from build123d import *

# Parameters (mm, degrees)
F1_DEPTH = 76.2
F3_DEPTH = 27.94
F4_R     = 10.16
F5_DEPTH = 76.201
F6_W     = 5.08
F6_H     = 76.2
F7_DEPTH = 10.16
F8_R     = 14.139528
F9_DEPTH = 25.4


with BuildPart() as f1:
    # F0 (on Right) → F1 (new body)
    with BuildSketch(Plane.YZ):
        Polygon((-76.2, 35.56), (-76.2, 0), (35.56, 0), (71.12, 35.56), (71.12, 71.12), (35.56, 71.12), (0, 35.56), align=None)
    extrude(amount=F1_DEPTH)

    # F2 (on face) → F3 (cut)
    with BuildSketch(Plane.XY.offset(71.12)):
        with BuildLine():
            Line((60.96, 60.96), (15.24, 60.96))
            ThreePointArc((15.24, 60.96), (7.62, 53.34), (15.24, 45.72))
            Line((15.24, 45.72), (60.96, 45.72))
            ThreePointArc((60.96, 45.72), (68.58, 53.34), (60.96, 60.96))
        make_face()
    extrude(amount=-F3_DEPTH, mode=Mode.SUBTRACT)

    # F4 (on face) → F5 (cut, through all)
    with BuildSketch(Plane.YZ.offset(76.2)):
        with Locations((17.78, 20.32)):
            Circle(F4_R)
    extrude(amount=-F5_DEPTH, mode=Mode.SUBTRACT)

    # F6 (on face) → F7 (cut)
    with BuildSketch(Plane.XY.offset(35.56)):
        with Locations((36.052045, -38.1)):
            Rectangle(F6_W, F6_H)
    extrude(amount=-F7_DEPTH, mode=Mode.SUBTRACT)

    # F8 (on face) → F9 (cut)
    with BuildSketch(Plane.XY.offset(35.56)):
        with Locations((36.461484, -37.369102)):
            Circle(F8_R)
    extrude(amount=-F9_DEPTH, mode=Mode.SUBTRACT)


solid = f1.part
The listing builds one solid part. Answer for the finished solid, in the listing's coordinates (mm). A direction names the side the tool comes from. Coordinates: 2 decimals unless noted, no trailing zeros. Order: outer loops, then holes, each group sorted by start corner. A loop starts at its lowest first (then second) coordinate and runs counter-clockwise, first axis right, second up. Notation, with made-up numbers: (20, 18) -> (26, 18) arc R30 ccw to (26, 57) -> close; hole circle Ø2 at (17.5, 35.25). An arc over 180 degrees is marked (long way). Answer in a Markdown table with one row per item. Add a question column.
Item 1: Find section C-C (z = 20.32). Write down the section's boundary in (x, y).
Item 2: Each of these flat-tipped pins is pushed along its axis until it touches: P1, Ø5.5, axis at x = 35.5, y = -17.5, coming from the +Z side; P2, Ø2.5, axis at x = 36, y = -60.5, coming from the +Z side; P3, Ø2, axis at x = 13.5, z = 23.5, coming from the +Y side. Where does it stop, or does it pass through?
Item 3: Find section D-D (x = 20). Write down the section's boundary in (y, z), then the cut area to 3 significant figures.
Item 4: Which of the six approach directions +Z, -Z, +X, -X, +Y, -Y give full straight-line access (tool end or side, diameter ignored) to faces 5 (the face through (37.57, 53.09, 17.53)), 6 (the face through (38, -21, 0)), 7 (the face through (33.512, -64, 31)), 8 (the face through (36, -37, 10.16)), 9 (the face through (17, -38, 35.56))?
Item 5: Find section B-B (z = 49). Write down the section's boundary in (x, y), then the cut area to 3 significant figures.
Item 6: Find the intervals of material crossed by L1, parallel to Y at x = 36.5, z = 25; L2, parallel to Y at x = 39.5, z = 22.5; L3, parallel to X at y = -9, z = 27, in increasing order. Write a range as from..to.
Item 7: Find section A-A (y = 17.78). Write down the section's boundary in (x, z).
Item 8: Determine the mould class of faces 1 (the face through (33.512, -12, 31)), 2 (the face through (38, -76.2, 18)), 3 (the face through (76.2, -4, 28)), 4 (the face through (0, -4, 28)) for opening direction X: +X half, -X half, draft (parallel to the pull), parting line (faces both ways), or undercut.
Result set:
| question | item | result |
|---|---|---|
| 1 | outline | (0, -76.2) -> (76.2, -76.2) -> (76.2, 7.62) -> (0, 7.62) -> close; (0, 27.94) -> (76.2, 27.94) -> (76.2, 55.88) -> (0, 55.88) -> close; hole circle Ø28.28 at (36.46, -37.37) |
| 2 | P1 | stops at z = 35.56 |
| 2 | P2 | stops at z = 25.4 |
| 2 | P3 | stops at y = 60.06 |
| 3 | outline | (-76.2, 0) -> (35.56, 0) -> (71.12, 35.56) -> (71.12, 71.12) -> (60.96, 71.12) -> (60.96, 43.18) -> (45.72, 43.18) -> (45.72, 71.12) -> (35.56, 71.12) -> (0, 35.56) -> (-76.2, 35.56) -> close; hole circle Ø20.32 at (17.78, 20.32) |
| 3 | area | 5,750 mm² |
| 4 | face 5 | -Z, +X, -X, +Y |
| 4 | face 6 | -Z, +X, -X, +Y, -Y |
| 4 | face 7 | +Z, -Y |
| 4 | face 8 | +Z |
| 4 | face 9 | +Z, +X, -X, -Y |
| 5 | outline | (0, 13.44) -> (76.2, 13.44) -> (76.2, 71.12) -> (0, 71.12) -> close; hole (15.24, 45.72) -> (60.96, 45.72) arc R7.62 ccw to (60.96, 60.96) -> (15.24, 60.96) arc R7.62 ccw to start |
| 5 | area | 3,520 mm² |
| 6 | L1 | y = -76.2..-51.51, -23.23..8.76, 26.8..60.56 |
| 6 | L2 | y = -76.2..-51.18, -23.56..7.86, 27.7..58.06 |
| 6 | L3 | x = 0..33.51, 38.59..76.2 |
| 7 | outline | (0, 0) -> (76.2, 0) -> (76.2, 10.16) -> (0, 10.16) -> close; (0, 30.48) -> (76.2, 30.48) -> (76.2, 53.34) -> (0, 53.34) -> close |
| 8 | face 1 | undercut |
| 8 | face 2 | draft |
| 8 | face 3 | +X half |
| 8 | face 4 | -X half |
